Part model, mm, in its own coordinate system. A direction names the side the tool comes from. Give positions to 0.01 mm unless a question says otherwise; leave off trailing zeros. Order: outer loops, then holes, each group sorted by start corner. A loop starts at its lowest first (then second) coordinate and runs counter-clockwise, first axis right, second up. Notation, with made-up numbers: M 6.5,-20.75 L 24.5,-20.75 A18 ccw 24.5,-9.75 Z; hole C 80,-15 d10. An arc over 180 degrees is marked long. Return JSON: item names as keys, results as strings.
Autodesk Fusion 360 part; units mm, degrees
sketch "Sketch1" plane through (0, 0, 0) normal (0, 0, 1) x (1, 0, 0)
  line L0 (135, 141) -> (-135, 141)
  line L1 (-135, 141) -> (-135, -141)
  line L2 (-135, -141) -> (135, -141)
  line L3 (135, -141) -> (135, 141)
  line L4 (135, 141) -> (-135, -141) construction
  line L5 (-135, 141) -> (135, -141) construction
  line L6 (-104.0059, 123) -> (104.0059, 123)
  line L7 (104, -108.6222) -> (-104, -108.6222)
  line L8 (-116, 111.3778) -> (-104.0059, 123)
  line L9 (-116, -96.6222) -> (-116, 111.3778)
  line L10 (-116, 121.1556) -> (-116, 123.3778)
  line L11 (0, 86.9957) -> (0, -79.0579) construction
  line L12 (116, 111.3778) -> (104.0059, 123)
  line L13 (116, 123.3776) -> (116, 121.1556)
  line L14 (116, 111.3778) -> (116, -96.6222)
  line L15 (-116, -96.6222) -> (-104, -108.6222)
  line L16 (104, -108.6222) -> (116, -96.6222)
  circle A0 centre (-114.5, -110) radius 2.2479
  circle A1 centre (114.5, -110) radius 2.2479
  dimension "d1" = 270
  dimension "d2" = 282
  dimension "d3" = 232
  dimension "d5" = 18
  dimension "d6" = 19
  dimension "d7" = 12
  dimension "d8" = 12
  dimension "d13" = 4.4958
  dimension "d14" = 4.4958
  dimension "d15" = 229
  dimension "d16" = 31
  dimension "d17" = 20.5
extrude "Extrude1" add sketch "Sketch1" along normal blind 3.1
chamfer "Chamfer1" distance 20 angle 45 2 edges at (135, 141, 1.55) (-135, 141, 1.55)
chamfer "Chamfer2" distance 2.286 angle 45 2 edges at (112.4042, -109.1871, 0) (-116.5958, -109.1871, 0)
equation "d6 = ( ( 270 - 232 ) / 2 ) * 1 mm"
equation "d17 = ( ( 270 - 229 ) / 2 ) * 1 mm"
Q1. Two-plate mould, pull along X, no slides. Class faces 1 (the flat face through (125, 131, 2)), 2 (the flat face through (-110.08, -102.54, 1.53)), 3 (the flat face through (118, 2, 0)): +X half, -X half, draft (parallel to the pull), parting line (faces both ways), or undercut.
Established:
{"face 1": "+X half", "face 2": "undercut", "face 3": "draft"}
Q2. Band-saw the part on B-B (y = 16.5). Give the cut face in (x, z), then the cut area to 3 significant figures.
Established:
{"outline": "M -135,0 L -116,0 L -116,3.1 L -135,3.1 Z; M 116,0 L 135,0 L 135,3.1 L 116,3.1 Z", "area": "118 mm²"}
Q3. 3-axis set-ups, long thin cutter, end or side, ignore diameter. For faces 4 (the flat face through (-125, 131, 2)), 5 (the flat face through (-110.087, 117.108, 1.528)): which of +Z, -Z, +X, -X, +Y, -Y reach the whole face in a straight line?
Established:
{"face 4": "+Z, -Z, -X, +Y", "face 5": "+Z, -Z"}
Q4. Band-saw the part on A-A (x = -20). Give the cut face in (y, z), then the cut area to 3 significant figures.
Established:
{"outline": "M -141,0 L -108.62,0 L -108.62,3.1 L -141,3.1 Z; M 123,0 L 141,0 L 141,3.1 L 123,3.1 Z", "area": "156 mm²"}
Q5. Band-saw the part on C-C (z = 1.4). Give the cut face in (x, y).
Established:
{"outline": "M -135,-141 L 135,-141 L 135,121 L 115,141 L -115,141 L -135,121 Z; hole C -114.5,-110 d6.27; hole M -116,-96.62 L -104,-108.62 L 104,-108.62 L 116,-96.62 L 116,111.38 L 104.01,123 L -104.01,123 L -116,111.38 Z; hole C 114.5,-110 d6.27"}
Q6. Probe line 1 along Y through (x, z) = (-101, 2.7); line 2 along X through (y, z) = (-46, 1.25); line 3 along X through (y, z) = (-112, 0.6). List the from-to ranges inside material, lowest first.
Established:
{"line 1": "y = -141 to -108.62, 123 to 141", "line 2": "x = -135 to -116, 116 to 135", "line 3": "x = -135 to -117.89, -111.11 to 111.11, 117.89 to 135"}
